For this review, take the finished solid that the model builds, in its own axes (mm). A direction names the side the tool comes from. Give positions to 0.01 mm unless a question says otherwise; leave off trailing zeros. Write each loop counter-clockwise with the first axis right and the second up, starting at its lowest first coordinate (ties: lowest second). Pieces come first, ordered by that corner, then holes.
1) For P1, Ø5, axis at x = -13, z = -3.5, coming from the -Y side; P2, Ø3, axis at x = 1, z = -1.5, coming from the +Y side, all flat-tipped, find the tip position at first contact; note any pin that passes through.
2) Wall thickness on line 1 along X through (y, z) = (27.5, 3); line 2 along X through (y, z) = (9, -4); line 3 along X through (y, z) = (6.25, -3) (3 decimals): over which ranges is each line inside the solid? List them lowest first.
3) We need section C-C on z = -3.75. Give the boundary of the cut face in (x, y).
4) Draft analysis for pull direction X (two halves, no side actions). For faces 1 (the face through (0, 15, -5)), 2 (the face through (17.605, 5.07, 0.07)), 3 (the face through (35, 15, 0)), state which applies: pulls with the +X half, pulls with the -X half, needs draft (parallel to the pull), parting line crosses it, or undercut.
5) We need section B-B on y = 22.5. Give the boundary of the cut face in (x, z).
6) We need section A-A on y = 2.5. Give the boundary of the cut face in (x, z), and give its area (3 significant figures).
7) We need section D-D on x = 2. Give the boundary of the cut face in (y, z).
8) Machinability: for faces 4 (the face through (-5, 25, 0)), 5 (the face through (-17.605, 5.07, 0.07)), 6 (the face through (20, 30, 0)), which of the approach directions +Z, -Z, +X, -X, +Y, -Y give a long, thin tool a straight path to every point of the face, cutting with its end or side? Answer none if there is none.
Autodesk Fusion 360 part; units mm, degrees
sketch "Sketch1" plane through (0, 0, 0) normal (0, 1, 0) x (1, 0, 0)
  line L0 (35, -5) -> (-35, -5)
  line L1 (-35, -5) -> (-35, 5)
  line L2 (-35, 5) -> (35, 5)
  line L3 (35, 5) -> (35, -5)
  line L4 (35, -5) -> (-35, 5) construction
  line L5 (-35, -5) -> (35, 5) construction
  dimension "d1" = 70
  dimension "d2" = 10
extrude "Extrude1" add sketch "Sketch1" along normal blind 30
sketch "Sketch2" plane through (0, 0, 5) normal (0, 0, 1) x (1, 0, 0)
  line L0 (-35, 0) -> (35, 0)
  line L1 (35, 0) -> (35, 30)
  line L2 (35, 30) -> (-35, 30)
  line L3 (-35, 30) -> (-35, 0)
  line L4 (0, 30) -> (-5, 30)
  line L5 (0, 30) -> (5, 30)
  line L6 (-25, 0) -> (-25, 10)
  line L7 (-25, 10) -> (-10, 0)
  line L8 (25, 0) -> (25, 10)
  line L9 (25, 10) -> (10, 0)
  line L10 (-25, 0) -> (-10, 0)
  line L11 (10, 0) -> (25, 0)
  line L12 (-5, 30) -> (-5, 20)
  line L13 (-5, 20) -> (5, 20)
  line L14 (5, 20) -> (5, 30)
  line L15 (-35, 30) -> (-35, 0)
  line L16 (-25, 0) -> (-35, 0)
  line L17 (-35, 30) -> (35, 30)
  line L18 (35, 30) -> (35, 0)
  line L19 (35, 0) -> (-10, 0)
  dimension "d5" = 5
  dimension "d6" = 5
  dimension "d7" = 10
  dimension "d8" = 10
  dimension "d9" = 10
  dimension "d10" = 15
  dimension "d13" = 10
extrude "Extrude2" cut sketch "Sketch2" against normal blind 10 contours L0 L6 L7 L10 | L2 L4 L5 L12 L13 L14 L17 | L0 L8 L9 L11 L19
Results list:
1. P1: stops at y = 0.33
1. P2: stops at y = 20
2. line 1: x = -35 to -5, 5 to 35
2. line 2: x = -35 to -25, -23.5 to 23.5, 25 to 35
2. line 3: x = -35 to -25, -19.375 to 19.375, 25 to 35
3. outline: (-35, 0) - (-25, 0) - (-25, 10) - (-10, 0) - (10, 0) - (25, 10) - (25, 0) - (35, 0) - (35, 30) - (5, 30) - (5, 20) - (-5, 20) - (-5, 30) - (-35, 30) - close
4. face 1: needs draft
4. face 2: undercut
4. face 3: pulls with the +X half
5. outline: (-35, -5) - (-5, -5) - (-5, 5) - (-35, 5) - close; (5, -5) - (35, -5) - (35, 5) - (5, 5) - close
6. outline: (-35, -5) - (-25, -5) - (-25, 5) - (-35, 5) - close; (-13.75, -5) - (13.75, -5) - (13.75, 5) - (-13.75, 5) - close; (25, -5) - (35, -5) - (35, 5) - (25, 5) - close
6. area: 475 mm2
7. outline: (0, -5) - (20, -5) - (20, 5) - (0, 5) - close
8. face 4: +Z, -Z, +Y
8. face 5: +Z, -Z, -Y
8. face 6: +Z, -Z, +X, -X, +Y
